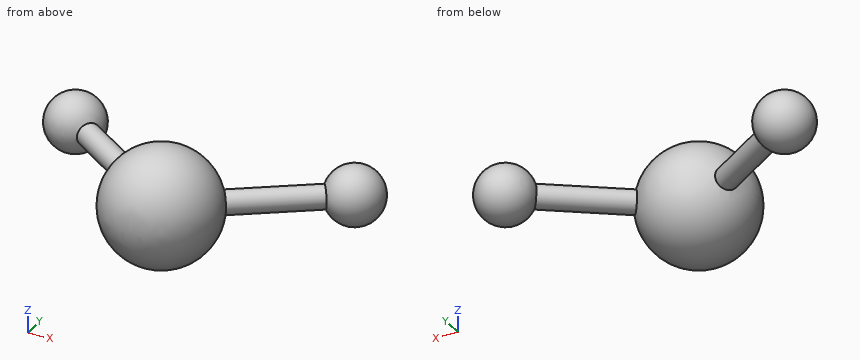
from build123d import *

# Parameters (mm, degrees)
F6_COUNT  = 2
F6_ANGLE  = 109.5
F8_R      = 1.27
F9_DEPTH  = 19.03992
F10_COUNT = 2
F10_ANGLE = 109.5


with BuildPart() as f2:
    # F1 (on Top) → F2 (revolve)
    with BuildSketch(Plane.XY):
        with BuildLine():
            Line((6.35, 0), (-6.35, 0))
            ThreePointArc((-6.35, 0), (0, -6.35), (6.35, 0))
        make_face()
    revolve(axis=Axis((0, 0, 0), (1, 0, 0)))



with BuildPart() as f4:
    # F3 (on Top) → F4 (revolve)
    with BuildSketch(Plane.XY):
        with BuildLine():
            Line((-12.3820216258, 10.9946158702), (-18.7320216258, 10.9946158702))
            ThreePointArc((-18.7320216258, 10.9946158702), (-15.5570216258, 7.8196158702), (-12.3820216258, 10.9946158702))
        make_face()
    revolve(axis=Axis((-15.5570216258, 10.9946158702, 0), (1, 0, 0)))


with BuildPart() as f6_1:
    # F6: instance of F4
    add(f4.part.rotate(Axis((0, 0, 9.7665896936), (0, 0, -1)), 1 * F6_ANGLE / (F6_COUNT - 1)))


with BuildPart() as f2_1:
    add(f2.part)

    add(f6_1.part)  # F9 merges F6_1
    # F8 (on line) → F9 (join)
    with BuildSketch(Plane(origin=(0, 0, 0), x_dir=(-0.57714519, 0.8166415552, 0), z_dir=(0.8166415552, 0.57714519, 0))):
        Circle(F8_R)
    extrude(amount=F9_DEPTH)



with BuildPart() as f2_2:
    add(f2_1.part)

    add(f4.part)  # F10 merges F4
    # F10: F2 ×2 about axis
    f10_axis = Axis((0, 0, 9.7665896936), (0, 0, 1))
    for i in range(1, F10_COUNT):
        add(f2_1.part.rotate(f10_axis, i * F10_ANGLE / (F10_COUNT - 1)))


solid = f2_2.part
The model under review builds one solid part; all positions refer to its coordinate system, in mm. Round coordinates to 2 decimals unless told otherwise and drop trailing zeros. Write each loop counter-clockwise with the first axis right and the second up, starting at its lowest first coordinate (ties: lowest second). Pieces come first, ordered by that corner, then holes. Notation, with made-up numbers: (-6, 75) -> (34, 75) arc R31 ccw to (34, 100) -> close; hole circle Ø7 at (48, 7.25). An arc over 180 degrees is marked (long way). Answer as a JSON object with one key per item and string values.
1. We need section C-C on z = -0.5. State the section outline as (x, y) points.
Results found:
{"outline": "(-13.85, 8.36) -> (-5.75, 2.64) arc R6.33 ccw (long way) to (5.75, 2.64) -> (13.85, 8.36) arc R3.14 ccw (long way) to (12.51, 10.27) -> (4.41, 4.54) arc R6.33 ccw to (-4.41, 4.54) -> (-12.51, 10.27) arc R3.14 ccw (long way) to start"}
2. We need section D-D on x = 3. State the section outline as (y, z) points.
Results found:
{"outline": "circle Ø11.19 at (0, 0)"}
3. We need section A-A on z = 2.75. State the section outline as (x, y) points, and give its area (3 significant figures).
Results found:
{"outline": "circle Ø3.17 at (-15.56, 10.99); circle Ø11.45 at (0, 0); circle Ø3.17 at (15.56, 10.99)", "area": "119 mm^2"}
4. We need section B-B on y = 13.25. State the section outline as (x, z) points.
Results found:
{"outline": "circle Ø4.47 at (-15.56, 0); circle Ø4.47 at (15.56, 0)"}
5. Clearance check with flat-ended pins moving along their axes: pin 1 (5 mm diameter, centred on x = -4, z = -1, fed in from -Y); pin 2 (4 mm diameter, centred on y = 8, z = 0.5, fed in from -X); pin 3 (6 mm diameter, centred on x = 7, z = 0.5, fed in from +Y). State where each tip first meets the part, or that it passes through.
Results found:
{"pin 1": "stops at y = -6.14", "pin 2": "stops at x = -18.56", "pin 3": "stops at y = 8.6"}
6. To check wall thickness, follow line 1 along Z through (x, y) = (1, -3); line 2 along Y through (x, z) = (4, -3.25); line 3 along Y through (x, z) = (-16.5, 2). State the ranges of each line that lie inside material, in increasing order.
Results found:
{"line 1": "z = -5.51 to 5.51", "line 2": "y = -3.71 to 3.71", "line 3": "y = 8.72 to 13.27"}
